from build123d import *

# Parameters (mm, degrees)
F1_DEPTH = 30
F2_R     = 1.5


with BuildPart() as f1:
    # F0 (on Top) → F1 (new body)
    with BuildSketch(Plane.XY):
        with BuildLine():
            ThreePointArc((7.009619, 22.5), (7.009619, 7.5), (20, 0))
            Line((20, 0), (68.038476, 0))
            ThreePointArc((68.038476, 0), (81.028857, 7.5), (81.028857, 22.5))
            Line((81.028857, 22.5), (57.009619, 64.10254))
            ThreePointArc((57.009619, 64.10254), (44.019238, 71.60254), (31.028857, 64.10254))
            Line((31.028857, 64.10254), (7.009619, 22.5))
        make_face()
        with BuildLine():
            Line((11.339746, 20), (35.358984, 61.60254))
            ThreePointArc((35.358984, 61.60254), (44.019238, 66.60254), (52.679492, 61.60254))
            Line((52.679492, 61.60254), (76.69873, 20))
            ThreePointArc((76.69873, 20), (76.69873, 10), (68.038476, 5))
            Line((68.038476, 5), (20, 5))
            ThreePointArc((20, 5), (11.339746, 10), (11.339746, 20))
        make_face(mode=Mode.SUBTRACT)
    extrude(amount=F1_DEPTH)

    # F2
    f2_edges = [f1.edges().sort_by_distance(p)[0] for p in [
        (31.028857, 64.10254, 15),
        (7.009619, 22.5, 15),
        (19.019238, 43.30127, 0),
        (19.019238, 43.30127, 30),
        (11.339746, 20, 15),
        (35.358984, 61.60254, 15),
        (23.349365, 40.80127, 0),
        (23.349365, 40.80127, 30),
    ]]
    fillet(f2_edges, radius=F2_R)


solid = f1.part
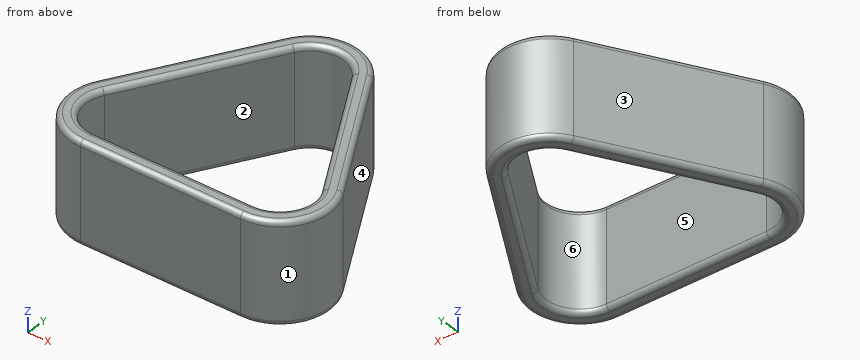
Here's how the part is built. I have some questions about the finished solid (model axes, mm). Face numbers are marked on the shaded views. A direction names the side the tool comes from. Round coordinates to 2 decimals unless told otherwise and drop trailing zeros. Write each loop counter-clockwise with the first axis right and the second up, starting at its lowest first coordinate (ties: lowest second). Pieces come first, ordered by that corner, then holes.
1. For the marked faces 1 and 2, which set-ups out of +Z, -Z, +X, -X, +Y, -Y let a thin tool reach every point of the face, with its end or its side?
2. Suppose I cut it at A-A (z = 16.5). List the corners of the cut face in (x, y) for me.
3. Will these pins go through, and if not, where does the flat tip stop? pin 1 Ø4 at (y, z) = (44, 16.5) entering from +X; pin 2 Ø1 at (y, z) = (45, 11) entering from -X; pin 3 Ø4 at (y, z) = (8, 6) entering from -X.
4. If we mould it in two halves opening along X, with no side actions, what happens to the marked faces 3, 4, 5 and 6? For each: released by +X, released by -X, zero draft, split by the parting line, or undercut.
5. I need wall thicknesses on L1, parallel to X at y = 15, z = 5; L2, parallel to Y at x = 33, z = 23; L3, parallel to Y at x = 60.5, z = 13.5. Which ranges of each line are inside material? Lowest first, please.
Answer sheet:
1. face 1: +Z, -Z, +X
1. face 2: +Z, -Z
2. outline: (7.01, 22.5) arc R15 ccw to (20, 0) - (68.04, 0) arc R15 ccw to (81.03, 22.5) - (57.01, 64.1) arc R15 ccw to (31.03, 64.1) - close; hole (11.34, 20) arc R10 ccw to (20, 5) - (68.04, 5) arc R10 ccw to (76.7, 20) - (52.68, 61.6) arc R10 ccw to (35.36, 61.6) - close
3. pin 1: stops at x = 69.77
3. pin 2: stops at x = 19.71
3. pin 3: stops at x = 5.86
4. face 3: released by -X
4. face 4: released by +X
4. face 5: undercut
4. face 6: undercut
5. L1: x = 5 to 10, 78.04 to 83.04
5. L2: y = 0 to 5, 57.52 to 66.78
5. L3: y = 0 to 5, 48.06 to 58.06
